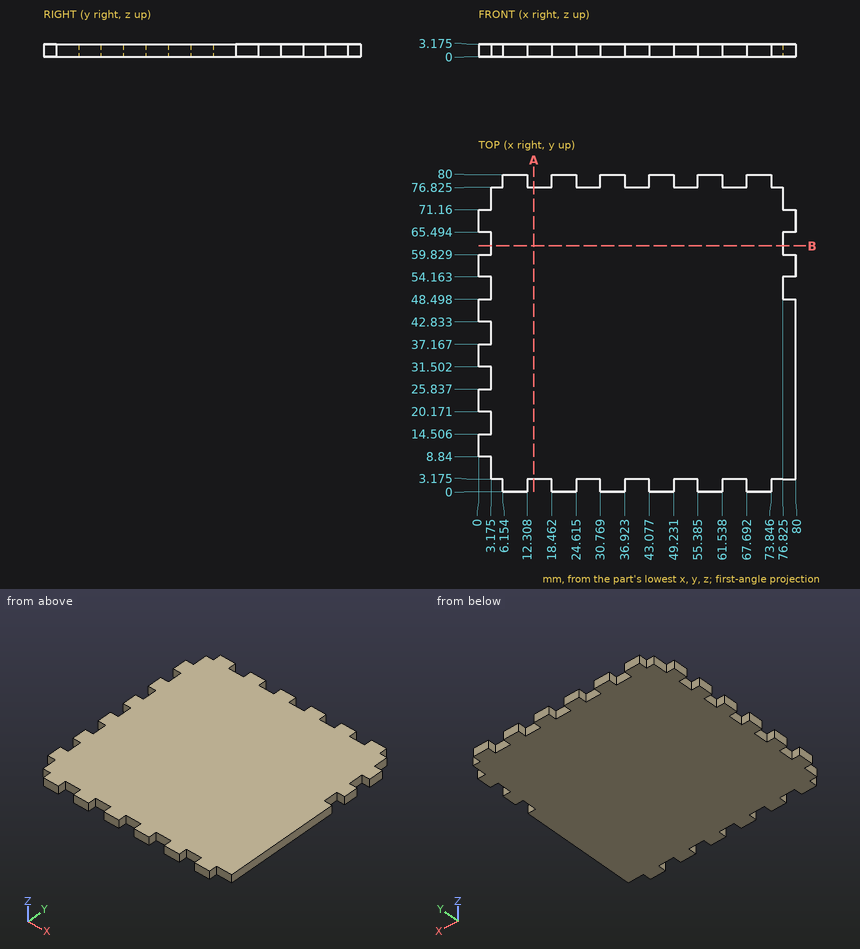
Could you check a few things on this drawing? It's one solid part, dimensions in mm from its lowest x, y, z. Coordinates: 2 decimals unless noted, no trailing zeros. Loops run counter-clockwise (first coordinate to the right, second up) from the corner with the lowest first, then second, coordinate; pieces in that order, holes last. Notation, with made-up numbers: (35.5, -29) - (42.5, -29) arc R19 cw to (42.5, -7) - close; hole circle Ø4 at (-19.5, 54). An arc over 180 degrees is marked (long way). Answer as a JSON object with one key per item and string values. Group by question number.
Item 1: If we section it at A-A (x = 14): List the corners of the cut face in (y, z) for me (1 decimal).
Item 2: For pin 1 (1 mm diameter, centred on x = 19.5, y = 59, fed in from -Z); pin 2 (1.6 mm diameter, centred on y = 1.5, z = 2, fed in from +X); pin 3 (1.6 mm diameter, centred on y = 78.5, z = 1, fed in from -X); pin 4 (1.6 mm diameter, centred on x = 27.5, z = 1, fed in from -Y) (3 decimals), each with a flat end and sliding along its axis, tell me the tip position at first contact or that it passes through.
Item 3: If I drill on L1, parallel to X at y = 8.5, z = 0.7 (1 decimal); L2, parallel to Y at x = 55, z = 1.4 (1 decimal), over which ranges is the centre line in solid material (lowest first)? Write a range as from..to.
Returned:
{
 "1": {"outline": "(3.2, 0) - (76.8, 0) - (76.8, 3.2) - (3.2, 3.2) - close"},
 "2": {"pin 1": "stops at z = 0", "pin 2": "stops at x = 73.85", "pin 3": "stops at x = 6.15", "pin 4": "stops at y = 3.175"},
 "3": {"L1": "x = 3.2..80", "L2": "y = 3.2..76.8"}
}
